```python
from build123d import *

# Parameters (mm, degrees)
SENSOR_HEIGHT_DEPTH               = 9
SENSOR_LIP_HEIGHT_DEPTH           = 2
SHORT_SIDE_EDGE_ROUNDING_R        = 5
SENSOR_HOLES_R                    = 1
EXTRUDED_SENSOR_HOLES_DEPTH       = 26.880736079
BOTTOM_TRIANGLE_CUT_DEPTH         = 1.5
TOP_TRIANGLE_CUT_DEPTH            = 1.5
FILAMENT_HOLE_CUT_DEPTH           = 2.5
FILAMENT_PROFILE_R                = 0.175
SENSING_START                     = -2
SENSING_FILAMENT_R                = 0.175
SENSING_FILAMENT_R_2              = 0.15
SENSING_PORTION_OF_FILAMENT_DEPTH = 2


# Read off the part's stored shape, not the designer's step: Sensor Lip Height
with BuildPart() as part:
    # Basic Sensor Dimensions → Sensor Height (new body)
    with BuildSketch(Plane.XY):
        with BuildLine():
            Line((-21.5, 8), (-21.5, -8))
            Line((-21.5, -8), (8.5, -11.25))
            ThreePointArc((8.5, -11.25), (19.75, 0), (8.5, 11.25))
            Line((8.5, 11.25), (-21.5, 8))
        make_face()
    extrude(amount=SENSOR_HEIGHT_DEPTH)

    # Sensor Lip Height outline → Sensor Lip Height (add)
    with BuildSketch(Plane.XY):
        with BuildLine():
            ThreePointArc((9.375, -11.215920604), (21.5, 0), (9.375, 11.215920604))
            ThreePointArc((9.375, 11.215920604), (19.75, 0), (9.375, -11.215920604))
        make_face()
    extrude(amount=SENSOR_LIP_HEIGHT_DEPTH)

    # Short Side Edge Rounding
    short_side_edge_rounding_edges = [part.edges().sort_by_distance(p)[0] for p in [
        (-21.5, -8, 4.5),
        (-21.5, 8, 4.5),
    ]]
    fillet(short_side_edge_rounding_edges, radius=SHORT_SIDE_EDGE_ROUNDING_R)

    # Sensor Holes → Extruded Sensor Holes (cut, through all)
    with BuildSketch(Plane.XY.offset(9)):
        with Locations((-16.044332748, -8.591030619)):
            Circle(SENSOR_HOLES_R)
        with Locations((-13.044332748, -8.916030619)):
            Circle(SENSOR_HOLES_R)
        with Locations((-10.044332748, -9.241030619)):
            Circle(SENSOR_HOLES_R)
        with Locations((-7.044332748, -9.566030619)):
            Circle(SENSOR_HOLES_R)
        with Locations((-10.044332748, 9.241030619)):
            Circle(SENSOR_HOLES_R)
        with Locations((-7.044332748, 9.566030619)):
            Circle(SENSOR_HOLES_R)
        with Locations((-13.044332748, 8.916030619)):
            Circle(SENSOR_HOLES_R)
        with Locations((-16.044332748, 8.591030619)):
            Circle(SENSOR_HOLES_R)
    extrude(amount=-EXTRUDED_SENSOR_HOLES_DEPTH, mode=Mode.SUBTRACT)

    # Bottom Triangle → Bottom Triangle Cut (cut)
    with BuildSketch(Plane(origin=(-1.106012767, -10.209348617, 0), x_dir=(0.9941830955390242, -0.10770316868339427, 0), z_dir=(-0.10770316868339427, -0.9941830955390242, 0))):
        with BuildLine():
            Line((6.91221696, 1.5), (6.91221696, 9))
            Line((6.91221696, 9), (6.16221696, 9))
            Line((6.16221696, 9), (6.41221696, 1.790726708))
            add(Edge.make_bspline(
                [(6.41221696, 1.790726708), (6.66221696, 1.5), (6.91221696, 1.5)],
                knots=[0, 0, 0, 0.5, 0.5, 0.5], degree=2))
        make_face()
        with BuildLine():
            Line((7.41221696, 1.790726708), (7.66221696, 9))
            Line((7.66221696, 9), (6.91221696, 9))
            Line((6.91221696, 9), (6.91221696, 1.5))
            add(Edge.make_bspline(
                [(6.91221696, 1.5), (7.16221696, 1.5), (7.41221696, 1.790726708)],
                knots=[0.5, 0.5, 0.5, 1, 1, 1], degree=2))
        make_face()
    extrude(amount=-BOTTOM_TRIANGLE_CUT_DEPTH, mode=Mode.SUBTRACT)

    # Top Triangle → Top Triangle Cut (cut)
    with BuildSketch(Plane(origin=(-1.106012767, 10.209348617, 0), x_dir=(0.9941830955390242, 0.10770316868339432, 0), z_dir=(-0.10770316868339432, 0.9941830955390242, 0))):
        with BuildLine():
            Line((6.91221696, -9), (7.66221696, -9))
            Line((7.66221696, -9), (7.41221696, -1.790726708))
            add(Edge.make_bspline(
                [(6.91221696, -1.5), (7.16221696, -1.5), (7.41221696, -1.790726708)],
                knots=[0.5, 0.5, 0.5, 1, 1, 1], degree=2))
            Line((6.91221696, -1.5), (6.91221696, -9))
        make_face()
        with BuildLine():
            Line((6.16221696, -9), (6.91221696, -9))
            Line((6.91221696, -9), (6.91221696, -1.5))
            add(Edge.make_bspline(
                [(6.41221696, -1.790726708), (6.66221696, -1.5), (6.91221696, -1.5)],
                knots=[0, 0, 0, 0.5, 0.5, 0.5], degree=2))
            Line((6.41221696, -1.790726708), (6.16221696, -9))
        make_face()
    extrude(amount=-TOP_TRIANGLE_CUT_DEPTH, mode=Mode.SUBTRACT)

    # Filament Hole → Filament Hole Cut (cut)
    with BuildSketch(Plane(origin=(0, 0, 0), x_dir=(-1, 0, 0), z_dir=(0, 0, -1))):
        with BuildLine():
            Line((4.5, 1), (1.5, 1))
            Line((1.5, 1), (1.5, -1))
            Line((1.5, -1), (4.5, -1))
            ThreePointArc((4.5, -1), (5.5, 0), (4.5, 1))
        make_face()
    extrude(amount=-FILAMENT_HOLE_CUT_DEPTH, mode=Mode.SUBTRACT)

    # Filament: sweep along a curve in space
    with BuildLine() as filament_path:
        Line((-3.5, 0, 0), (-3.5, 0, 2.5))
        Line((-3.5, 0, 0), (5.692388155, 0, -9.192388155))
    # Filament profile (on start of the path) → Filament (sweep)
    with BuildSketch(Plane(origin=(5.692388155, 0, -9.192388155), x_dir=(0.7071067811865488, 0, 0.7071067811865464), z_dir=(-0.7071067811865464, 0, 0.7071067811865488))):
        Circle(FILAMENT_PROFILE_R)
    sweep(path=filament_path.line, transition=Transition.RIGHT)

    # Sensing Filament → Sensing Portion of Filament (cut)
    with BuildSketch(Plane(origin=(7.442388155, 0, -7.442388155), x_dir=(-0.7071067811865488, 0, -0.7071067811865462), z_dir=(0.7071067811865462, 0, -0.7071067811865488)).offset(SENSING_START)):
        with Locations((2.474873734, 0)):
            Circle(SENSING_FILAMENT_R)
        with Locations((2.474873734, 0)):
            Circle(SENSING_FILAMENT_R_2, mode=Mode.SUBTRACT)
    extrude(amount=SENSING_PORTION_OF_FILAMENT_DEPTH, mode=Mode.SUBTRACT)


solid = part.part
```
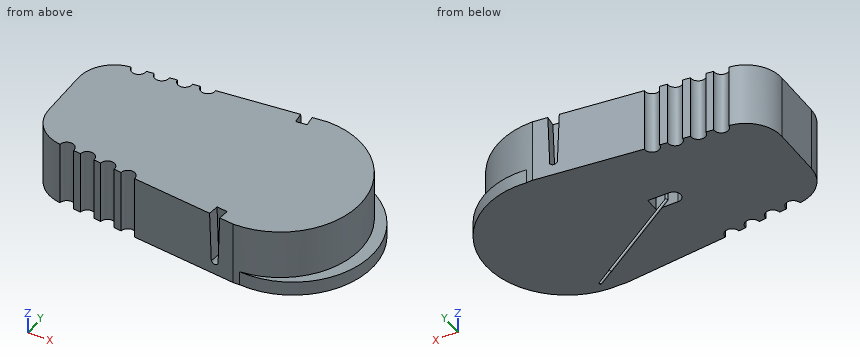
Check sheet for the modelled part. Datum: model origin and axes. Units: mm. Give positions to 0.01 mm unless a question says otherwise; leave off trailing zeros. Write each loop counter-clockwise with the first axis right and the second up, starting at its lowest first coordinate (ties: lowest second). Pieces come first, ordered by that corner, then holes.
Item 1: Cross-section at D-D (y = -5). Enter the section's corners in (x, z), and give its area (3 significant figures).
Item 2: Cross-section at A-A (z = 0.5). Enter the section's corners in (x, y) (3 decimals).
Item 3: Scan lines: L1, parallel to Z at x = 11.5, y = -1; L2, parallel to X at y = 9.25, z = 2.75; L3, parallel to Y at x = 15.5, z = 3.25. Record each from-to range of solid material in increasing order.
Item 4: Gauge pin test, flat ends, axial feed: pin 1 (6 mm diameter, centred on y = 2, z = -6.5, fed in from +X); pin 2 (2 mm diameter, centred on x = -3.5, z = 1, fed in from -Y); pin 3 (0.6 mm diameter, centred on x = -4, y = -0.5, fed in from -Z). Record the tip position at first contact, or that the pin passes through.
Item 5: Cross-section at B-B (y = -2). Enter the section's corners in (x, z), and give its area (3 significant figures).
Item 6: Cross-section at C-C (x = 14). Enter the section's corners in (y, z).
Report:
1. outline: (-21.27, 0) - (20.33, 0) - (20.33, 2) - (18.58, 2) - (18.58, 9) - (-21.27, 9) - close
1. area: 362 mm2
2. outline: (-21.5, -3.512) arc R5 ccw to (-17.039, -8.483) arc R1 cw to (-15.05, -8.699) - (-14.039, -8.808) arc R1 cw to (-12.05, -9.024) - (-11.039, -9.133) arc R1 cw to (-9.05, -9.349) - (-8.039, -9.458) arc R1 cw to (-6.05, -9.674) - (8.5, -11.25) arc R11.25 ccw to (9.375, -11.216) arc R11.25 ccw (long way) to (9.375, 11.216) arc R11.25 ccw to (8.5, 11.25) - (-6.05, 9.674) arc R1 cw to (-8.039, 9.458) - (-9.05, 9.349) arc R1 cw to (-11.039, 9.133) - (-12.05, 9.024) arc R1 cw to (-14.039, 8.808) - (-15.05, 8.699) arc R1 cw to (-17.039, 8.483) arc R5 ccw to (-21.5, 3.512) - close; circle Ø0.35 at (-3.5, 0); hole (-4.5, -1) - (-1.5, -1) - (-1.5, 1) - (-4.5, 1) arc R1 ccw to start
3. L1: z = 0 to 9
3. L2: x = -9.04 to -7.99, -6.1 to 14.9
3. L3: y = -8.81 to 8.81
4. pin 1: stops at x = 5.48
4. pin 2: stops at y = -10.06
4. pin 3: stops at z = 2.5
5. outline: (-21.5, 0) - (21.32, 0) - (21.32, 2) - (19.57, 2) - (19.57, 9) - (-21.5, 9) - close
5. area: 373 mm2
6. outline: (-10.61, 0) - (10.61, 0) - (10.61, 2) - (9.81, 2) - (9.81, 9) - (-9.81, 9) - (-9.81, 2) - (-10.61, 2) - close
